The listing builds one solid part. Answer for the finished solid, in the listing's coordinates (mm). A direction names the side the tool comes from. Round coordinates to 2 decimals unless told otherwise and drop trailing zeros. Write each loop counter-clockwise with the first axis right and the second up, starting at its lowest first coordinate (ties: lowest second). Pieces come first, ordered by that corner, then holes. Notation, with made-up numbers: (16, 86.5) - (24, 86.5) arc R29 ccw to (24, 121.5) - close; hole circle Ø6 at (11.25, -33.5). An arc over 180 degrees is marked (long way). Return JSON: item names as keys, results as strings. Group by question number.
from build123d import *

# Parameters (mm, degrees)
F0_W      = 135
F0_H      = 90
F0_R      = 1.75
F0_W_2    = 120
F0_H_2    = 77
F1_DEPTH  = 2
F2_DEPTH  = 18
F3_R      = 2.25
F4_DEPTH  = 25
F5_DEPTH  = 1.5
F7_DEPTH  = 143.001
F8_W      = 12
F8_H      = 18
F9_DEPTH  = 3.5
F10_R     = 2.25
F11_DEPTH = 3.501
F12_R     = 2.25
F13_DEPTH = 3.501
F14_W     = 135
F14_H     = 2.5
F15_DEPTH = 2.5


# Not quite as in the source:
# - a feature names something its author has since deleted; it is built from what else it names


with BuildPart() as f1:
    # F0 (on Front) → F1 (new body)
    with BuildSketch(Plane.XZ):
        with Locations((41.872507602, -14.5468179137)):
            Rectangle(F0_W, F0_H)
        with Locations((-21.627492398, -49.7468179137)):
            Circle(F0_R, mode=Mode.SUBTRACT)
        with Locations((105.872507602, -49.7468179137)):
            Circle(F0_R, mode=Mode.SUBTRACT)
        with Locations((-21.627492398, 20.8531820863)):
            Circle(F0_R, mode=Mode.SUBTRACT)
        with Locations((42.122507602, -14.4468179137)):
            Rectangle(F0_W_2, F0_H_2, mode=Mode.SUBTRACT)
        with Locations((105.872507602, 20.8531820863)):
            Circle(F0_R, mode=Mode.SUBTRACT)
    extrude(amount=F1_DEPTH)

    # F0 (on Front) → F2 (join)
    with BuildSketch(Plane.XZ):
        Polygon((-25.627492398, -59.5468179137), (-25.627492398, 30.4531820863), (-29.627492398, 30.4531820863), (-29.627492398, -64.5468179137), (113.372507602, -64.5468179137), (113.372507602, 30.4531820863), (109.372507602, 30.4531820863), (109.372507602, -59.5468179137), align=None)
    extrude(amount=F2_DEPTH)

    # F3 (on face) → F4 (cut)
    with BuildSketch(Plane(origin=(0, 0, -64.5468179137), x_dir=(1, 0, 0), z_dir=(0, 0, -1))):
        with Locations((-9.627492398, 9)):
            Circle(F3_R)
        with Locations((41.872507602, 9)):
            Circle(F3_R)
        with Locations((93.372507602, 9)):
            Circle(F3_R)
    extrude(amount=-F4_DEPTH, mode=Mode.SUBTRACT)

    # F5 (cut): a face of the model
    f5_faces = [f1.faces().sort_by_distance(p)[0] for p in [
        (41.872507602, -3.3594484176, -59.5468179137),
    ]]
    extrude(f5_faces, amount=-F5_DEPTH, mode=Mode.SUBTRACT)

    # F6 (on face) → F7 (cut, through all)
    with BuildSketch(Plane.YZ.offset(113.372507602)):
        with BuildLine():
            Line((-18, 30.4531820863), (-18, -54.0468179137))
            Line((-18, -54.0468179137), (-9.6275595227, -54.0468179137))
            ThreePointArc((-9.6275595227, -54.0468179137), (-6.7891073566, -53.1630284647), (-4.9540928207, -50.8240936338))
            ThreePointArc((-4.9540928207, -50.8240936338), (-4.6144653792, -49.6089954864), (-4.5, -48.3525290189))
            Line((-4.5, -48.3525290189), (-4.5, 30.4531820863))
            Line((-4.5, 30.4531820863), (-18, 30.4531820863))
        make_face()
    extrude(amount=-F7_DEPTH, mode=Mode.SUBTRACT)

    # F8 (on face) → F9 (join, through all)
    with BuildSketch(Plane(origin=(0, 0, -64.5468179137), x_dir=(1, 0, 0), z_dir=(0, 0, -1))):
        with Locations((-35.627492398, 9)):
            Rectangle(F8_W, F8_H)
        with Locations((119.372507602, 9)):
            Rectangle(F8_W, F8_H)
    extrude(amount=-F9_DEPTH)

    # F10 (on face) → F11 (cut, through all)
    with BuildSketch(Plane.XY.offset(-61.0468179137)):
        with Locations((-36.627492398, -9)):
            Circle(F10_R)
        with Locations((120.372507602, -9)):
            Circle(F10_R)
    extrude(amount=-F11_DEPTH, mode=Mode.SUBTRACT)

    # F12 (on face) → F13 (cut, through all)
    with BuildSketch(Plane.XY.offset(-61.0468179137)):
        with BuildLine():
            Line((34.372507602, -4), (-14.4826919802, -4))
            ThreePointArc((-14.4826919802, -4), (-17.4280077943, -4.959565029), (-19.2428347866, -7.4699540979))
            Line((-19.2428347866, -7.4699540979), (-22.627492398, -18))
            Line((-22.627492398, -18), (106.372507602, -18))
            Line((106.372507602, -18), (102.9878499906, -7.4699540979))
            ThreePointArc((102.9878499906, -7.4699540979), (101.1730229983, -4.959565029), (98.2277071842, -4))
            Line((98.2277071842, -4), (49.372507602, -4))
            Line((49.372507602, -4), (49.372507602, -9))
            ThreePointArc((49.372507602, -9), (41.872507602, -16.5), (34.372507602, -9))
            Line((34.372507602, -9), (34.372507602, -4))
        make_face()
        with Locations((-9.627492398, -9)):
            Circle(F12_R, mode=Mode.SUBTRACT)
        with Locations((93.372507602, -9)):
            Circle(F12_R, mode=Mode.SUBTRACT)
    extrude(amount=-F13_DEPTH, mode=Mode.SUBTRACT)

    # F14 (on face) → F15 (join)
    with BuildSketch(Plane.XY.offset(30.4531820863)):
        with Locations((41.872507602, -3.25)):
            Rectangle(F14_W, F14_H)
        Polygon((-29.627492398, -4.5), (-25.627492398, -4.5), (-25.627492398, -2), (109.372507602, -2), (109.372507602, -4.5), (113.372507602, -4.5), (113.372507602, 0), (-29.627492398, 0), align=None)
    extrude(amount=F15_DEPTH)


solid = f1.part
(1) Find section B-B (x = 11.5). Write down the section's boundary in (y, z).
(2) Find section C-C (y = -14.5). Write down the section's boundary in (x, z), plus the area to 3 significant figures.
(3) Find section A-A (z = -18). Write down the section's boundary in (x, y).
(4) Determine the mould class of faces 5 (the flat face through (-41.627, -9, -63)), 6 (the flat face through (42, -4.5, 31)), 7 (the flat face through (10, -4, -63)) for opening direction X: +X half, -X half, draft (parallel to the pull), parting line (faces both ways), or undercut.
(5) For faces 1 (the flat face through (74, -4, -63)), 2 (the cylindrical face through (107.49, -0.99, -50.42)), 3 (the flat face through (-34, -9, -61.047)), 4 (the flat face through (111, -14, -54.047)), determine the directions among +Z, -Z, +X, -X, +Y, -Y from which every point of the face is accessible in a straight line to the end or side of a thin tool.
(6) Consider line 1 (X direction, y = -3.75, z = -57.5); line 2 (Z direction, x = 17, y = -1); line 3 (Y direction, x = -28, z = -33). Determine where each line is inside the solid, lowest interval first.
(7) Flat-ended cylindrical pins translate along their axes: pin 1 (8 mm diameter, centred on x = 41, y = -8.5, fed in from -Z); pin 2 (8 mm diameter, centred on y = -7.5, z = 7.5, fed in from -X); pin 3 (1 mm diameter, centred on y = -0.5, z = -31.5, fed in from +X); pin 4 (3.5 mm diameter, centred on x = 41.87, y = -9, fed in from -Z). Find the tip coordinate at first contact, or state that the pin passes through.
Check sheet entries:
{
 "1": {"outline": "(-4.5, 30.45) - (-2, 30.45) - (-2, 24.05) - (0, 24.05) - (0, 32.95) - (-4.5, 32.95) - close; (-4, -64.55) - (0, -64.55) - (0, -52.95) - (-2, -52.95) - (-2, -61.05) - (-4, -61.05) - close"},
 "2": {"outline": "(-41.63, -64.55) - (-21.5, -64.55) - (-21.5, -61.05) - (-25.63, -61.05) - (-25.63, -54.05) - (-29.63, -54.05) - (-29.63, -61.05) - (-41.63, -61.05) - close; (36.77, -64.55) - (46.97, -64.55) - (46.97, -61.05) - (36.77, -61.05) - close; (105.25, -64.55) - (125.37, -64.55) - (125.37, -61.05) - (113.37, -61.05) - (113.37, -54.05) - (109.37, -54.05) - (109.37, -61.05) - (105.25, -61.05) - close", "area": "233 mm^2"},
 "3": {"outline": "(-29.63, -4.5) - (-25.63, -4.5) - (-25.63, -2) - (-17.88, -2) - (-17.88, 0) - (-29.63, 0) - close; (102.12, -2) - (109.37, -2) - (109.37, -4.5) - (113.37, -4.5) - (113.37, 0) - (102.12, 0) - close"},
 "4": {"face 5": "-X half", "face 6": "draft", "face 7": "undercut"},
 "5": {"face 1": "-Z, -Y", "face 2": "+Y, -Y", "face 3": "+Z, -X, +Y, -Y", "face 4": "+Z, +X, -X, -Y"},
 "6": {"line 1": "x = -29.63 to -25.63, 109.37 to 113.37", "line 2": "z = -64.55 to -52.95, 24.05 to 32.95", "line 3": "y = -4.5 to 0"},
 "7": {"pin 1": "stops at z = -64.55", "pin 2": "stops at x = -29.63", "pin 3": "stops at x = 113.37", "pin 4": "passes through"}
}
